Geometry check sheet. Reference: the model listing, model coordinates, mm. A direction names the side the tool comes from. Give positions to 0.01 mm unless a question says otherwise; leave off trailing zeros. Order: outer loops, then holes, each group sorted by start corner. A loop starts at its lowest first (then second) coordinate and runs counter-clockwise, first axis right, second up. Notation, with made-up numbers: M 39.5,0.25 L 90.5,0.25 A15 ccw 90.5,19.25 Z; hole C -21.5,-37.75 d4. An arc over 180 degrees is marked long. Put each result on its own line as item: value. Start each with the question number.
Q1. Section check A-A on y = 40. Record the cut outline in (x, z), then the cut area to 3 significant figures.
Q2. Material ranges on L1, parallel to Y at x = 0, z = -13.25; L2, parallel to X at y = 35.5, z = -4; L3, parallel to Z at x = -39, y = 36.5, recorded low to high.
Q3. Section check D-D on y = 9. Record the cut outline in (x, z), then the cut area to 3 significant figures.
Q4. Mould release check, pull along X, two halves, no side actions. Record for faces 4 (the flat face through (-50, 17, -23)), 5 (the flat face through (1, 20, -36)), 6 (the flat face through (50, 17, -23)), 7 (the flat face through (0, 10, -40)): +X half, -X half, draft (parallel to the pull), parting line (faces both ways), or undercut.
Q5. Section check B-B on x = 0. Record the cut outline in (y, z).
Q6. Go/stop test with flat-tipped pins: pin 1 (10 mm diameter, centred on x = 7.5, y = 34, fed in from -Z); pin 2 (20 mm diameter, centred on x = 8, z = -35, fed in from +Y); pin 3 (6 mm diameter, centred on x = -11.5, y = 5.5, fed in from -Z). Record where each tip stops, or that it passes through.
Q7. Section check C-C on x = -33. Record the cut outline in (y, z), then the cut area to 3 significant figures.
Q8. Access from +Z, -Z, +X, -X, +Y, -Y to the whole of each face (thin tool, end or side, straight path). Record for faces 1 (the flat face through (30, 10, -50)), 2 (the flat face through (1, 0, -23)), 3 (the flat face through (12, 40, -20)).
```python
from build123d import *

# Parameters (mm, degrees)
BOSS_EXTRUDE1_DEPTH = 50
SKETCH2_R           = 10
CUT_EXTRUDE1_DEPTH  = 21
CUT_EXTRUDE2_REACH  = 22
SKETCH3_W           = 60
SKETCH3_H           = 20


with BuildPart() as part:
    # Sketch1 → Boss-Extrude1 (new body, symmetric)
    with BuildSketch(Plane(origin=(0, 0, 0), x_dir=(0, 0, -1), z_dir=(1, 0, 0))):
        Polygon((0, 0), (60, 0), (60, 20), (20, 20), (20, 60), (0, 60), align=None)
    extrude(amount=BOSS_EXTRUDE1_DEPTH, both=True)

    # Sketch2 → Cut-Extrude1 (cut, through all)
    with BuildSketch(Plane(origin=(0, 0, -20), x_dir=(-1, 0, 0), z_dir=(0, 0, -1))):
        with Locations((0, 40)):
            Circle(SKETCH2_R)
    extrude(amount=-CUT_EXTRUDE1_DEPTH, mode=Mode.SUBTRACT)

    # Sketch3 → Cut-Extrude2 (cut, up to next)
    with BuildSketch(Plane(origin=(0, 20, 0), x_dir=(1, 0, 0), z_dir=(0, 1, 0)), mode=Mode.PRIVATE) as cut_extrude2_sk1:
        with Locations((0, 50)):
            Rectangle(SKETCH3_W, SKETCH3_H)
    cut_extrude2_tool1 = extrude(cut_extrude2_sk1.sketch, amount=-CUT_EXTRUDE2_REACH, mode=Mode.PRIVATE) & part.part
    add(cut_extrude2_tool1.solids().sort_by_distance((0, 20, -50))[0], mode=Mode.SUBTRACT)


solid = part.part
```
Results found:
1. outline: M -50,-20 L -10,-20 L -10,0 L -50,0 Z; M 10,-20 L 50,-20 L 50,0 L 10,0 Z
1. area: 1,600 mm^2
2. L1: y = 0 to 30, 50 to 60
2. L2: x = -50 to -8.93, 8.93 to 50
2. L3: z = -20 to 0
3. outline: M -50,-60 L -30,-60 L -30,-40 L 30,-40 L 30,-60 L 50,-60 L 50,0 L -50,0 Z
3. area: 4,800 mm^2
4. face 4: -X half
4. face 5: draft
4. face 6: +X half
4. face 7: undercut
5. outline: M 0,-40 L 20,-40 L 20,-20 L 30,-20 L 30,0 L 0,0 Z; M 50,-20 L 60,-20 L 60,0 L 50,0 Z
6. pin 1: stops at z = -20
6. pin 2: stops at y = 20
6. pin 3: stops at z = -40
7. outline: M 0,-60 L 20,-60 L 20,-20 L 60,-20 L 60,0 L 0,0 Z
7. area: 2,000 mm^2
8. face 1: -Z, +Y, -Y
8. face 2: +Z, -Z, +X, -X, -Y
8. face 3: -Z, +X, -X, +Y
